```python
from build123d import *

# Parameters (mm, degrees)
SKETCH1_R           = 28.575
EXTRUDE1_DEPTH      = 27.0002
EXTRUDE1_DEPTH_BACK = 84.1248
CUT_EXTRUDE1_REACH  = 86.125
SKETCH2_R           = 28.575
SKETCH2_R_2         = 23.622
CUT_EXTRUDE3_START  = -27.0002
CUT_EXTRUDE3_DEPTH  = 27.0002
SKETCH18_R          = 9.525
CUT_EXTRUDE4_DEPTH  = 0.254
SKETCH19_R          = 9.525
CUT_EXTRUDE5_DEPTH  = 0.254
CHAMFER1_SIZE       = 0.762
SKETCH15_R          = 6.9469
EXTRUDE2_DEPTH      = 1.27
CIRPATTERN1_COUNT   = 4


with BuildPart() as part:
    # Sketch1 → Extrude1 (new body, two sides)
    with BuildSketch(Plane(origin=(0, 0, 0), x_dir=(0, 0, -1), z_dir=(1, 0, 0))) as extrude1_sk:
        Circle(SKETCH1_R)
    extrude(amount=EXTRUDE1_DEPTH)
    extrude(extrude1_sk.sketch, amount=-EXTRUDE1_DEPTH_BACK)

    # Sketch2 → Cut-Extrude1 (cut, up to next)
    with BuildSketch(Plane(origin=(0, 0, 0), x_dir=(0, 0, -1), z_dir=(1, 0, 0)), mode=Mode.PRIVATE) as cut_extrude1_sk1:
        Circle(SKETCH2_R)
        with Locations((0, -4.191)):
            Circle(SKETCH2_R_2, mode=Mode.SUBTRACT)
    cut_extrude1_tool1 = extrude(cut_extrude1_sk1.sketch, amount=-CUT_EXTRUDE1_REACH, mode=Mode.PRIVATE) & part.part
    add(cut_extrude1_tool1.solids().sort_by_distance((0, 0, 27.766777))[0], mode=Mode.SUBTRACT)

    # Sketch4 → Cut-Extrude3 (cut)
    with BuildSketch(Plane.ZY.offset(CUT_EXTRUDE3_START)):
        with BuildLine():
            Line((23.6855, -25.666178421), (23.6855, 17.476089577))
            Line((23.6855, 17.476089577), (0, 31.150919378))
            Line((0, 31.150919378), (-23.6855, 17.476089577))
            Line((-23.6855, 17.476089577), (-23.6855, -25.666178421))
            ThreePointArc((-23.6855, -25.666178421), (0, 34.925), (23.6855, -25.666178421))
        make_face()
    extrude(amount=CUT_EXTRUDE3_DEPTH, mode=Mode.SUBTRACT)

    # Sketch6 → Cut-Revolve2 (revolve, cut)
    with BuildSketch(Plane.XY, mode=Mode.PRIVATE) as cut_revolve2_sk:
        Polygon((0.750392661, 57.15), (27.0002, 11.684), (27.0002, 57.15), align=None)
    revolve(cut_revolve2_sk.sketch.rotate(Axis((-0.562097706, -4.191, 0), (1, 0, 0)), 270), axis=Axis((-0.562097706, -4.191, 0), (1, 0, 0)), mode=Mode.SUBTRACT)  # turned: the seam where the file's is

    # S2D0002 → Cut-Revolve3 (revolve, cut)
    with BuildSketch(Plane(origin=(9.0932, 23.136869081, 13.372742289), x_dir=(0, 0.5, -0.866025404), z_dir=(1, 0, 0))):
        Polygon((0, 0), (6.1849, 0), (5.642306865, -2.5527), (4.9784, -3.216606865), (4.9784, -13.462), (0, -13.462), align=None)
    revolve(axis=Axis((9.0932, 10.895513396, 6.305192289), (0, 0.866025404, 0.5)), mode=Mode.SUBTRACT)

    # Sketch8 → Cut-Revolve4 (revolve, cut)
    with BuildSketch(Plane(origin=(9.0932, 23.136869081, -13.372742289), x_dir=(0, -0.5, -0.866025404), z_dir=(1, 0, 0))):
        Polygon((0, 0), (6.1849, 0), (5.642306865, -2.5527), (4.9784, -3.216606865), (4.9784, -13.462), (0, -13.462), align=None)
    revolve(axis=Axis((9.0932, 10.895513396, -6.305192289), (0, 0.866025404, -0.5)), mode=Mode.SUBTRACT)

    # Sketch18 → Cut-Extrude4 (cut)
    with BuildSketch(Plane(origin=(0, 23.363189534, 13.488743766), x_dir=(1, 0, 0), z_dir=(0, 0.866025404, 0.5))):
        with Locations((9.0932, -0.0127)):
            Circle(SKETCH18_R)
    extrude(amount=-CUT_EXTRUDE4_DEPTH, mode=Mode.SUBTRACT)

    # Sketch19 → Cut-Extrude5 (cut)
    with BuildSketch(Plane(origin=(0, 23.363189534, -13.488743766), x_dir=(1, 0, 0), z_dir=(0, 0.866025404, -0.5))):
        with Locations((9.0932, 0.0127)):
            Circle(SKETCH19_R)
    extrude(amount=-CUT_EXTRUDE5_DEPTH, mode=Mode.SUBTRACT)

    # Sketch10 → Cut-Revolve6 (revolve, cut)
    with BuildSketch(Plane.XY, mode=Mode.PRIVATE) as cut_revolve6_sk:
        Polygon((0, 19.431), (0, 18.415), (-3.302, 18.415), (-4.318, 19.431), align=None)
    revolve(cut_revolve6_sk.sketch.rotate(Axis((-4.5339, -4.191, 0), (1, 0, 0)), 90), axis=Axis((-4.5339, -4.191, 0), (1, 0, 0)), mode=Mode.SUBTRACT)  # turned: the seam where the file's is

    # Sketch12 → Cut-Revolve8 (revolve, cut)
    with BuildSketch(Plane.XY, mode=Mode.PRIVATE) as cut_revolve8_sk:
        Polygon((-84.1248, 19.431), (-84.1248, 18.415), (-81.5848, 18.415), (-80.5688, 19.431), align=None)
    revolve(cut_revolve8_sk.sketch.rotate(Axis((-84.3026, -4.191, 0), (1, 0, 0)), 90), axis=Axis((-84.3026, -4.191, 0), (1, 0, 0)), mode=Mode.SUBTRACT)  # turned: the seam where the file's is

    # Chamfer1
    chamfer1_edges = [part.edges().sort_by_distance(p)[0] for p in [
        (-84.1248, -4.191, -22.606),
    ]]
    chamfer(chamfer1_edges, length=CHAMFER1_SIZE)

    # Sketch13 → Revolve1 (revolve)
    with BuildSketch(Plane(origin=(0, 0, 0), x_dir=(0, -1, 0), z_dir=(0, 0, 1)), mode=Mode.PRIVATE) as revolve1_sk:
        with BuildLine():
            Line((4.191, 27.0002), (4.191, 73.2028))
            Line((4.191, 73.2028), (14.2875, 73.2028))
            ThreePointArc((14.2875, 73.2028), (15.00592049, 72.90522049), (15.3035, 72.1868))
            Line((15.3035, 72.1868), (15.3035, 27.0002))
            Line((15.3035, 27.0002), (4.191, 27.0002))
        make_face()
    revolve(revolve1_sk.sketch.rotate(Axis((25.10663, -4.191, 0), (1, 0, 0)), 270), axis=Axis((25.10663, -4.191, 0), (1, 0, 0)))  # turned: the seam where the file's is

    # S2D0001 → Cut-Revolve9 (revolve, cut)
    with BuildSketch(Plane(origin=(64.8716, -9.9441, 0), x_dir=(0, -1, 0), z_dir=(0, 0, 1)), mode=Mode.PRIVATE) as cut_revolve9_sk:
        Polygon((0, 8.3312), (0, -8.6868), (-5.7531, -12.143611227), (-5.7531, 8.3312), align=None)
    revolve(cut_revolve9_sk.sketch.rotate(Axis((43.373048211, -4.191, 0), (1, 0, 0)), 270), axis=Axis((43.373048211, -4.191, 0), (1, 0, 0)), mode=Mode.SUBTRACT)  # turned: the seam where the file's is

    # Sketch15 → Extrude2 (add)
    with BuildSketch(Plane(origin=(27.0002, 23.143219081, -13.361743766), x_dir=(0, -0.5, -0.866025404), z_dir=(0, -0.866025404, 0.5))):
        with Locations((0.0127, -17.907)):
            Circle(SKETCH15_R)
    extrude(amount=-EXTRUDE2_DEPTH)

    # Sketch16 → Cut-Revolve10 (revolve, cut)
    with BuildSketch(Plane(origin=(60.9092, 3.666724106, -7.857724106), x_dir=(-1, 0, 0), z_dir=(0, -0.707106781, -0.707106781)), mode=Mode.PRIVATE) as cut_revolve10_sk:
        Polygon((-8.3312, 0), (-5.9182, 0), (-8.3312, -2.413), align=None)
    cut_revolve10 = revolve(cut_revolve10_sk.sketch.rotate(Axis((69.2404, 0.494324135, -4.685324135), (0, 0.707106781, -0.707106781)), 90), axis=Axis((69.2404, 0.494324135, -4.685324135), (0, 0.707106781, -0.707106781)), mode=Mode.SUBTRACT)  # turned: the seam where the file's is

    # CirPattern1: Cut-Revolve10 ×4 about axis
    cirpattern1_axis = Axis((25.10663, -4.191, 0), (-1, 0, 0))
    for i in range(1, CIRPATTERN1_COUNT):
        add(cut_revolve10.rotate(cirpattern1_axis, i * 360 / CIRPATTERN1_COUNT), mode=Mode.SUBTRACT)


solid = part.part
```
Geometry check sheet. Reference: the model listing, model coordinates, mm. A direction names the side the tool comes from. Round coordinates to 2 decimals unless told otherwise and drop trailing zeros. Order: outer loops, then holes, each group sorted by start corner. A loop starts at its lowest first (then second) coordinate and runs counter-clockwise, first axis right, second up. Notation, with made-up numbers: M 76,10.5 L 105,10.5 A19 ccw 105,16.5 Z; hole C 75.25,26.5 d1. An arc over 180 degrees is marked long. Write item = value, one per line.
Q1. Set-up check for faces 4 (the flat face through (9.024, 11.444, 6.702)), 5 (the flat face through (27, -7, 11)), 6 (the flat face through (16.13, 27.238, -6.777)): record each of +Z, -Z, +X, -X, +Y, -Y from which the full face is reachable in a straight line by a thin tool's end or side.
Answer block:
face_4 = none
face_5 = +X
face_6 = -Z, +X, +Y
Q2. Release check for a two-part mould opening along Z. For faces 1 (the cylindrical face through (49.277, 0.065, 10.265)), 2 (the conical face through (69.27, 2.88, 6.15)), 3 (the cylindrical face through (13.51, 14.704, -11.157)) record: released by +Z, released by -Z, zero draft, split by the parting line, or undercut.
Answer block:
face_1 = split by the parting line
face_2 = released by +Z
face_3 = undercut
Q3. Depth check by flat-ended pin: pin 1 Ø3 at (x, y) = (-65, -10) entering from +Z; pin 2 Ø3 at (x, z) = (-21, -5.5) entering from -Y; pin 3 Ø10 at (x, z) = (-16, 2.5) entering from +Y. Enter the tip coordinate at first touch or a pass-through.
Answer block:
pin_1 = 23.23
pin_2 = -27.47
pin_3 = 19.43
Q4. Scan lines: line 1 (X direction, y = 18, z = 10); line 2 (Y direction, x = 69, z = 0); line 3 (Y direction, x = -67, z = 0.5). Record each from-to range of solid material in increasing order.
Answer block:
line_1 = 0 to 4.13, 14.06 to 22.11
line_2 = -15.3 to -9.94, 1.56 to 6.92
line_3 = -27.81 to 19.43
Q5. Section check A-A (x = -31). Enter the section's corners in (y, z).
Answer block:
outline = C -4.19,0 d47.24
